Autodesk Inventor part; units mm, degrees
ref_plane "Work Plane1" through (10.3188, 0, 0) normal (-1, 0, 0) x (0, 0, 1)
ref_plane "YZ Plane" through (0, 0, 0) normal (1, 0, 0) x (0, 1, 0)
ref_plane "XZ Plane" through (0, 0, 0) normal (0, 1, 0) x (-1, 0, 0)
sketch "Sketch1" plane through (0, 0, 0) normal (0, 0, 1) x (1, 0, 0)
  line L0 (0, 0) -> (0, 3.1115)
  line L1 (0, 5.5562) -> (26.1938, 5.5563) construction
  line L2 (0, 7.9375) -> (26.1938, 7.9375) construction
  line L3 (26.1938, 7.9375) -> (26.1938, 5.5563) construction
  line L4 (26.1938, 5.5563) -> (26.1938, 0) construction
  line L5 (26.1938, 0) -> (24.6063, 0) construction
  line L6 (26.1938, 6.35) -> (34.3853, 6.35) construction
  line L7 (26.1938, 0) -> (34.3853, 0) construction
  line L8 (34.3853, 0) -> (34.3853, 6.35) construction
  line L9 (16.6688, 7.9375) -> (16.6688, 0) construction
  circle A0 centre (16.6688, 7.5565) radius 2.3813 construction
  circle A1 centre (16.6688, 5.4928) radius 2.3813 construction
  circle A2 centre (10.3188, 7.5565) radius 2.3813 construction
  circle A3 centre (10.3188, 5.4928) radius 2.3813 construction
  line L10 (10.3188, 7.9375) -> (10.3188, 0) construction
  line L11 (0, 5.1753) -> (8.7313, 5.1753) construction
  line L12 (8.7313, 5.1753) -> (8.7313, 0) construction
  line L13 (5.5563, 5.1753) -> (5.5563, 0) construction
  line L14 (18.2563, 5.1753) -> (18.2563, 0) construction
  line L15 (21.4313, 5.1753) -> (21.4313, 0) construction
  line L16 (0, 3.1115) -> (5.5563, 3.1115)
  line L17 (5.5563, 3.1115) -> (8.7313, 5.1753)
  line L18 (18.2563, 5.1753) -> (21.4313, 3.1115) construction
  line L19 (11.9063, 5.1753) -> (11.9063, 0) construction
  line L20 (15.0813, 5.1753) -> (15.0813, 0) construction
  line L21 (11.9063, 5.1753) -> (15.0813, 3.1115)
  line L22 (21.4313, 3.3734) -> (34.3853, 3.3734) construction
  line L23 (24.6063, 3.3734) -> (24.6063, 1.321) construction
  line L24 (21.4313, 3.3734) -> (20.1197, 5.5563) construction
  line L25 (26.1938, 3.1115) -> (30.9563, 3.1115) construction
  line L26 (30.9563, 3.1115) -> (30.9563, 0) construction
  line L27 (31.75, 3.3734) -> (31.75, 0) construction
  line L28 (31.75, 0) -> (29.723, 3.3734) construction
  line L29 (0, 7.9375) -> (-1.5875, 7.9375) construction
  line L30 (-1.5875, 7.9375) -> (-1.5875, 3.3734) construction
  line L31 (-1.5875, 3.3734) -> (5.5563, 3.3734) construction
  line L32 (5.5563, 3.1115) -> (15.0813, 3.1115) construction
  line L33 (15.0813, 3.1115) -> (23.5304, 3.1115)
  line L34 (11.9063, 5.1753) -> (26.1938, 5.1753) construction
  line L35 (8.7313, 5.1753) -> (11.9063, 5.1753)
  line L36 (24.6063, 3.1115) -> (26.1938, 3.1115) construction
  line L37 (24.6063, 1.321) -> (23.5304, 3.1115)
  line L38 (25.4, 0) -> (25.4, 3.3734) construction
  line L39 (24.6063, 1.321) -> (24.6063, 0)
  line L40 (23.5304, 3.1115) -> (24.6063, 3.1115) construction
  line L41 (0, 3.1115) -> (0, 12.7) construction
  line L42 (24.6063, 0) -> (0, 0)
  line L43 (24.6063, 1.321) -> (25.4, 0) construction
  point P0 (0, 0)
  dimension "d0" = 12.7
  dimension "d1" = 5.5563
  dimension "d2" = 7.9375
  dimension "d3" = 26.1938
  dimension "d4" = 8.1915
  dimension "d5" = 6.35
  dimension "d6" = 9.525
  dimension "d7" = 6.35
  dimension "d8" = 0.381
  dimension "d9" = 0.381
  dimension "d10" = 0.0635
  dimension "d11" = 0.0635
  dimension "d12" = 1.5875
  dimension "d13" = 4.7625
  dimension "d14" = 1.5875
  dimension "d15" = 4.7625
  dimension "d17" = 1.5875
  dimension "d18" = 4.7625
  dimension "d19" = 3.3734
  dimension "d20" = 3.175
  dimension "d21" = 31
  dimension "d23" = 9.525
  dimension "d24" = 0.7937
  dimension "d25" = 31
  dimension "d26" = 1.5875
  dimension "d33" = 4.7625
  dimension "d35" = 31
  dimension "d36" = 3.3734
  dimension "d37" = 3.1115
  dimension "d38" = 0.7937
  dimension "d43" = 10.3187
revolve "Revolution1" add sketch "Sketch1" angle 360 about axis through (24.6063, 0, 0) along (-1, 0, 0)
ref_plane "Work Plane1" through (10.3188, 0, 0) normal (-1, 0, 0) x (0, 0, 1)
fillet "Fillet1" radius 3.9688 4 edges at (5.5563, -3.1115, 0) (15.0813, -3.1115, 0) (11.9063, -5.1753, 0) (8.7313, -5.1753, 0)
sketch "Sketch2" plane through (0, 0, 0) normal (-1, 0, 0) x (0, 0, 1)
  circle A0 centre (0, 0) radius 3.1115
extrude "Extrusion1" add sketch "Sketch2" along normal blind 23.5394
sketch "Sketch3" plane through (0, 0, 0) normal (0, 0, 1) x (1, 0, 0)
  line L0 (-23.5394, 3.1115) -> (4.3798, 3.1115)
  arc A0 (4.3798, 3.1115) -> (6.5427, 3.7527) centre (4.3798, 7.0802) ccw
  line L1 (6.5427, 3.7527) -> (7.7448, 4.5341)
  arc A1 (9.9077, 5.1753) -> (7.7448, 4.5341) centre (9.9077, 1.2065) ccw
  line L2 (9.9077, 5.1753) -> (10.7298, 5.1753)
  arc A2 (12.8927, 4.5341) -> (10.7298, 5.1753) centre (10.7298, 1.2065) ccw
  line L3 (12.8927, 4.5341) -> (14.0948, 3.7527)
  arc A3 (14.0948, 3.7527) -> (16.2577, 3.1115) centre (16.2577, 7.0803) ccw
  line L4 (16.2577, 3.1115) -> (23.5304, 3.1115)
  circle A4 centre (7.5381, 9.9656) radius 2.3812
  line L5 (4.3798, 7.0802) -> (4.3798, 3.1115) construction
  line L6 (4.3798, 7.0802) -> (6.5427, 3.7527) construction
  line L7 (9.9077, 1.2065) -> (7.7448, 4.5341) construction
  line L8 (9.9077, 1.2065) -> (9.9077, 5.1753) construction
  line L9 (10.7298, 1.2065) -> (10.7298, 5.1753) construction
  line L10 (10.7298, 1.2065) -> (12.8927, 4.5341) construction
  line L11 (16.2577, 7.0803) -> (14.0948, 3.7527) construction
  line L12 (16.2577, 7.0803) -> (16.2577, 3.1115) construction
  line L13 (-5.9448, 5.4927) -> (4.3798, 5.4927)
  arc A5 (4.3798, 5.4927) -> (5.2449, 5.7492) centre (4.3798, 7.0802) ccw
  line L14 (7.7448, 4.5341) -> (6.4471, 6.5306) construction
  line L15 (5.2449, 5.7492) -> (6.4471, 6.5306)
  line L16 (9.9077, 5.1753) -> (9.9077, 7.5565) construction
  arc A6 (9.9077, 7.5565) -> (6.4471, 6.5306) centre (9.9077, 1.2065) ccw
  point P0 (0, 0)
  dimension "d45" = 4.7625
  dimension "d47" = 2.3813
  dimension "d49" = 2.3876
sketch "Sketch4" plane through (-23.5394, 0, 0) normal (-1, 0, 0) x (0, 0, 1)
  circle A0 centre (0, 0) radius 3.1115
  circle A1 centre (0, 0) radius 4.2545
  dimension "d50" = 8.509
extrude "Extrusion2" add sketch "Sketch4" against normal blind 1.5875
sketch "Sketch5" plane through (-23.5394, 0, 0) normal (-1, 0, 0) x (0, 0, 1)
  circle A0 centre (0, 0) radius 4.2545
  circle A1 centre (0, 0) radius 3.175
  dimension "d54" = 6.35
extrude "Extrusion3" add sketch "Sketch5" along normal blind 4.9784 contours A1
sketch "Sketch6" plane through (0, 0, 0) normal (0, 1, 0) x (-1, 0, 0)
  line L0 (28.5178, -3.175) -> (28.5178, 3.175)
  line L1 (23.5394, 3.175) -> (23.5394, -3.175)
  line L2 (23.5394, 3.175) -> (28.5178, 3.175)
  line L3 (23.5394, -3.175) -> (28.5178, -3.175)
  circle A0 centre (29.4322, 0) radius 0.7874
  line L4 (28.6448, 3.175) -> (28.6448, -3.175) construction
  line L5 (28.5178, 0) -> (29.4322, 0) construction
  line L6 (28.5178, 3.175) -> (28.6448, 3.175) construction
  line L7 (28.6448, -3.175) -> (28.5178, -3.175) construction
  line L8 (28.5178, 3.175) -> (31.0578, 3.175)
  line L9 (31.0578, 3.175) -> (31.0578, 0)
  line L10 (31.0578, -3.175) -> (28.5178, -3.175) construction
  line L11 (28.5178, 0) -> (31.0578, 0)
  line L12 (31.0578, 0) -> (31.0578, -3.175) construction
  line L13 (28.5178, 0) -> (28.5178, 3.175)
  point P0 (0, 0)
  point P1 (30.2196, 0)
  point P2 (28.6448, 0)
  dimension "d57" = 1.5748
  dimension "d58" = 0.127
  dimension "d60" = 2.54
sketch "Sketch7" plane through (-28.5178, 0, 0) normal (-1, 0, 0) x (0, 0, 1)
  circle A0 centre (0, 0) radius 3.175
extrude "Extrusion4" add sketch "Sketch7" along normal blind 2.54
extrude "Extrusion5" cut sketch "Sketch6" along normal through all both and the other way through all contours L11 A0 | A0 L11
equation "\"d1\" = d28"
equation "\"d2\" = d29"
equation "\"d8\" = d30"
equation "\"d9\" = d8"
equation "\"d10\" = d31"
equation "\"d11\" = d10"
equation "\"d17\" = d12"
equation "\"d18\" = d13"
equation "\"d23\" = d22"
equation "\"d25\" = d21"
equation "\"d35\" = d25"
equation "\"d44\" = -d43"
properties part number "Shifting Shaft" material "Steel"
Part model, mm, in its own coordinate system. A direction names the side the tool comes from. Round coordinates to 2 decimals unless told otherwise and drop trailing zeros. Order: outer loops, then holes, each group sorted by start corner. A loop starts at its lowest first (then second) coordinate and runs counter-clockwise, first axis right, second up. Notation, with made-up numbers: M 88,57 L 132,57 A29 ccw 132,77 Z; hole C 67.25,46.5 d5. An arc over 180 degrees is marked long. Answer in a Markdown table with one row per item. Add a question column.
Q1. Wall check: L1, parallel to X at y = 0.5, z = 0; L2, parallel to Z at x = -22, y = 2; L3, parallel to X at y = 2, z = 0. Give the ranges that are in metal, low to high. Write a range as from..to.
Q2. Cut at A-A on x = -9. Give the cut face in (y, z).
Q3. Mould opens along X. For faces 4 (the face through (19.95, -0.67, -3.04)), 5 (the face through (-8.6, 2.45, -1.92)), 6 (the face through (-23.539, -3, -2)) say: +X half, -X half, draft (parallel to the pull), parting line (faces both ways), or undercut.
Q4. Pin check, flat tips, straight feed: pin 1 (3 mm diameter, centred on x = 18.5, y = -0.5, fed in from -Z); pin 2 (3 mm diameter, centred on x = -16.5, y = -2, fed in from +Z); pin 3 (2 mm diameter, centred on x = -10, y = -3.5, fed in from -Z). Stop position of each tip, or through.
Q5. 3-axis set-ups, long thin cutter, end or side, ignore diameter. For faces 1 (the face through (24.606, 0, 0)), 2 (the face through (-21.952, -3, -2)), 3 (the face through (-27.2, 2.8, 1.5)): which of +Z, -Z, +X, -X, +Y, -Y reach the whole face in a straight line?
Established:
| question | item | result |
|---|---|---|
| 1 | L1 | x = -31.06..-30.22, -28.64..24.61 |
| 1 | L2 | z = -3.76..3.76 |
| 1 | L3 | x = -31.06..-30.22, -28.64..24.2 |
| 2 | outline | C 0,0 d6.22 |
| 3 | face 4 | draft |
| 3 | face 5 | undercut |
| 3 | face 6 | -X half |
| 4 | pin 1 | stops at z = -3.11 |
| 4 | pin 2 | stops at z = 3.07 |
| 4 | pin 3 | stops at z = -1.85 |
| 5 | face 1 | +Z, -Z, +X, +Y, -Y |
| 5 | face 2 | none |
| 5 | face 3 | -X |
